Read the model definition and answer for the solid it produces. Units are mm, in the model's axes. A direction names the side the tool comes from. Give positions to 0.01 mm unless a question says otherwise; leave off trailing zeros. Order: outer loops, then holes, each group sorted by start corner. A loop starts at its lowest first (then second) coordinate and runs counter-clockwise, first axis right, second up. Notation, with made-up numbers: (47.5, 5.25) - (79.5, 5.25) arc R22 ccw to (79.5, 29.25) - close; hole circle Ø6 at (83.5, 29.5). An arc over 180 degrees is marked (long way). Answer as CSV lines item,"result". Start each with the question number.
from build123d import *

# Parameters (mm, degrees)
BOSS_EXTRUDE1_DEPTH = 3.175
SKETCH2_R           = 6.2992
CUT_EXTRUDE1_DEPTH  = 2.54


with BuildPart() as part:
    # Sketch1 → Boss-Extrude1 (new body)
    with BuildSketch(Plane.XZ.offset(66.817157288)):
        with BuildLine():
            Line((26.467944946, -26.475), (26.467944946, -25.350260413))
            ThreePointArc((26.467944946, -25.350260413), (29.642944946, -16.95), (26.467944946, -8.549739587))
            Line((26.467944946, -8.549739587), (26.467944946, -7.425))
            Line((26.467944946, -7.425), (25.343205359, -7.425))
            ThreePointArc((25.343205359, -7.425), (16.942944946, -4.25), (8.542684533, -7.425))
            Line((8.542684533, -7.425), (7.417944946, -7.425))
            Line((7.417944946, -7.425), (7.417944946, -8.549739587))
            ThreePointArc((7.417944946, -8.549739587), (4.242944946, -16.95), (7.417944946, -25.350260413))
            Line((7.417944946, -25.350260413), (7.417944946, -26.475))
            Line((7.417944946, -26.475), (8.542684533, -26.475))
            ThreePointArc((8.542684533, -26.475), (16.942944946, -29.65), (25.343205359, -26.475))
            Line((25.343205359, -26.475), (26.467944946, -26.475))
        make_face()
    extrude(amount=-BOSS_EXTRUDE1_DEPTH)

    # Sketch2 → Cut-Extrude1 (cut)
    with BuildSketch(Plane.XZ.offset(66.817157288)):
        with Locations(Location((16.942944946, -16.95, 0), (0, 0, 270))):
            Circle(SKETCH2_R)
    extrude(amount=-CUT_EXTRUDE1_DEPTH, mode=Mode.SUBTRACT)


solid = part.part
(1) Flat-ended cylindrical pins translate along their axes: pin 1 Ø1.2 at (x, y) = (8, -65.5) entering from +Z; pin 2 Ø0.9 at (y, z) = (-65, -26) entering from -X; pin 3 Ø1.2 at (x, y) = (26, -65.5) entering from -Z (3 decimals). Find the tip coordinate at first contact, or state that the pin passes through.
(2) Section A-A, the plane z = -16.95 is taken. Write down the section's boundary in (x, y), and give its area (3 significant figures).
(3) Section C-C, the plane x = 15.5 is taken. Write down the section's boundary in (y, z), and give its area (3 significant figures).
(4) Section D-D, the plane z = -8 is taken. Write down the section's boundary in (x, y), and give its area (3 significant figures).
(5) Which of the six approach directions +Z, -Z, +X, -X, +Y, -Y give full straight-line access (tool end or side, diameter ignored) to faces 4 (the flat face through (26, -65, -26.475)), 5 (the flat face through (26, -65, -7.425)), 6 (the flat face through (8, -65, -26.475)), 7 (the flat face through (7.418, -65, -8)), 8 (the cylindrical face through (10.794, -65.565, -15.584))?
(6) Determine the mould class of faces 1 (the cylindrical face through (16.81, -65.25, -29.65)), 2 (the flat face through (17, -64.277, -17)), 3 (the flat face through (26.468, -65, -26)) for opening direction Z: released by +Z, released by -Z, zero draft, split by the parting line, or undercut.
(7) Section B-B, the plane y = -65.05 is taken. Write down the section's boundary in (x, z) (3 decimals).
(8) Straight lines are drawn through the part: line 1 (X direction, y = -66.3, z = -16.95); line 2 (X direction, y = -64.9, z = -17.25) (3 decimals); line 3 (Z direction, x = 26.25, y = -64.15) (3 decimals). For each, find the intervals that lie inside material, in ascending order. Write a range as [from, to].
Checks:
1,pin 1,"stops at z = -7.37"
1,pin 2,"stops at x = 7.42"
1,pin 3,"stops at z = -26.475"
2,outline,"(4.24, -66.82) - (10.64, -66.82) - (10.64, -64.28) - (23.24, -64.28) - (23.24, -66.82) - (29.64, -66.82) - (29.64, -63.64) - (4.24, -63.64) - close"
2,area,"48.6 mm²"
3,outline,"(-66.82, -29.57) - (-63.64, -29.57) - (-63.64, -4.33) - (-66.82, -4.33) - (-66.82, -10.82) - (-64.28, -10.82) - (-64.28, -23.08) - (-66.82, -23.08) - close"
3,area,"49.0 mm²"
4,outline,"(7.42, -66.82) - (26.47, -66.82) - (26.47, -63.64) - (7.42, -63.64) - close"
4,area,"60.5 mm²"
5,face 4,"-Z, +X, +Y, -Y"
5,face 5,"+Z, +X, +Y, -Y"
5,face 6,"-Z, -X, +Y, -Y"
5,face 7,"+Z, -X, +Y, -Y"
5,face 8,"-Y"
6,face 1,"released by -Z"
6,face 2,"undercut"
6,face 3,"zero draft"
7,outline,"(7.418, -26.475) - (8.543, -26.475) arc R12.7 ccw to (25.343, -26.475) - (26.468, -26.475) - (26.468, -25.35) arc R12.7 ccw to (26.468, -8.55) - (26.468, -7.425) - (25.343, -7.425) arc R12.7 ccw to (8.543, -7.425) - (7.418, -7.425) - (7.418, -8.55) arc R12.7 ccw to (7.418, -25.35) - close; hole circle Ø12.598 at (16.943, -16.95)"
8,line 1,"x = [4.24, 10.64], [23.24, 29.64]"
8,line 2,"x = [4.246, 10.651], [23.235, 29.639]"
8,line 3,"z = [-26.475, -7.425]"
